Geometry: final body of the model. Coordinates: model frame, mm. Give positions to 0.01 mm unless a question says otherwise; leave off trailing zeros. Order: outer loops, then holes, each group sorted by start corner. A loop starts at its lowest first (then second) coordinate and runs counter-clockwise, first axis right, second up. Notation, with made-up numbers: (24, 15) -> (35, 15) arc R28 cw to (35, 45) -> close; hole circle Ø7 at (73.5, 53). An arc over 180 degrees is marked (long way). One line per question, with ' | ' between items.
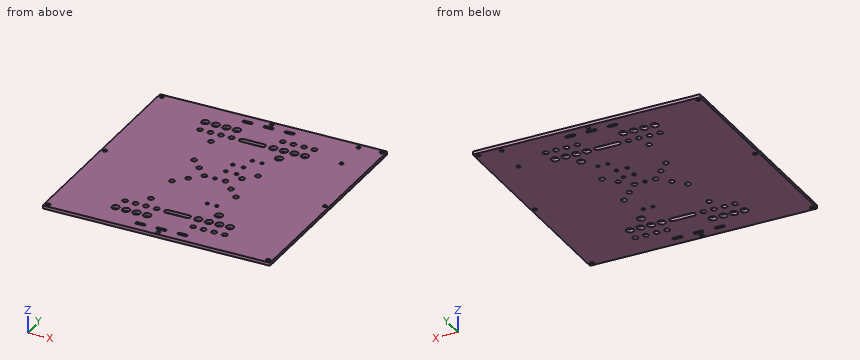
from build123d import *

# Parameters (mm, degrees)
SKETCH1_R           = 1.8
SKETCH1_R_2         = 2.5
SKETCH1_R_3         = 3.6
SKETCH1_R_4         = 1.57
SKETCH1_R_5         = 1.75
BOSS_EXTRUDE1_DEPTH = 3


with BuildPart() as part:
    # Sketch1 → Boss-Extrude1 (new body)
    with BuildSketch(Plane.XY):
        with BuildLine():
            Line((-107.125, -108), (107.125, -108))
            ThreePointArc((107.125, -108), (107.743718434, -107.743718434), (108, -107.125))
            Line((108, -107.125), (108, 107.125))
            ThreePointArc((108, 107.125), (107.743718434, 107.743718434), (107.125, 108))
            Line((107.125, 108), (-107.125, 108))
            ThreePointArc((-107.125, 108), (-107.743718434, 107.743718434), (-108, 107.125))
            Line((-108, 107.125), (-108, -107.125))
            ThreePointArc((-108, -107.125), (-107.743718434, -107.743718434), (-107.125, -108))
        make_face()
        with Locations((-104.5, -104.5)):
            Circle(SKETCH1_R, mode=Mode.SUBTRACT)
        with Locations((104.5, -104.5)):
            Circle(SKETCH1_R, mode=Mode.SUBTRACT)
        with Locations((-104.5, 104.5)):
            Circle(SKETCH1_R, mode=Mode.SUBTRACT)
        with Locations((104.5, 104.5)):
            Circle(SKETCH1_R, mode=Mode.SUBTRACT)
        with Locations((-49.85, -69)):
            Circle(SKETCH1_R_2, mode=Mode.SUBTRACT)
        with Locations((-39.85, -69)):
            Circle(SKETCH1_R_2, mode=Mode.SUBTRACT)
        with Locations((-29.85, -69)):
            Circle(SKETCH1_R_2, mode=Mode.SUBTRACT)
        with Locations((-19.855, -69)):
            Circle(SKETCH1_R_2, mode=Mode.SUBTRACT)
        with Locations((49.85, -69)):
            Circle(SKETCH1_R_3, mode=Mode.SUBTRACT)
        with Locations((39.85, -69)):
            Circle(SKETCH1_R_3, mode=Mode.SUBTRACT)
        with Locations((29.85, -69)):
            Circle(SKETCH1_R_3, mode=Mode.SUBTRACT)
        with Locations((19.855, -69)):
            Circle(SKETCH1_R_3, mode=Mode.SUBTRACT)
        with Locations((0, -104.5)):
            Circle(SKETCH1_R, mode=Mode.SUBTRACT)
        with Locations((0, 104.5)):
            Circle(SKETCH1_R, mode=Mode.SUBTRACT)
        with Locations((49.85, 69)):
            Circle(SKETCH1_R_3, mode=Mode.SUBTRACT)
        with Locations((39.85, 69)):
            Circle(SKETCH1_R_3, mode=Mode.SUBTRACT)
        with Locations((29.85, 69)):
            Circle(SKETCH1_R_3, mode=Mode.SUBTRACT)
        with Locations((19.855, 69)):
            Circle(SKETCH1_R_3, mode=Mode.SUBTRACT)
        with Locations((-19.855, 69)):
            Circle(SKETCH1_R_2, mode=Mode.SUBTRACT)
        with Locations((-29.85, 69)):
            Circle(SKETCH1_R_2, mode=Mode.SUBTRACT)
        with Locations((-39.85, 69)):
            Circle(SKETCH1_R_2, mode=Mode.SUBTRACT)
        with Locations((-49.85, 69)):
            Circle(SKETCH1_R_2, mode=Mode.SUBTRACT)
        with Locations((-104.5, 0)):
            Circle(SKETCH1_R, mode=Mode.SUBTRACT)
        with Locations((104.5, 0)):
            Circle(SKETCH1_R, mode=Mode.SUBTRACT)
        with Locations((-51.83, -82.65)):
            Circle(SKETCH1_R_3, mode=Mode.SUBTRACT)
        with Locations((-41.83, -82.65)):
            Circle(SKETCH1_R_3, mode=Mode.SUBTRACT)
        with Locations((-31.83, -82.65)):
            Circle(SKETCH1_R_3, mode=Mode.SUBTRACT)
        with Locations((-21.835, -82.65)):
            Circle(SKETCH1_R_3, mode=Mode.SUBTRACT)
        with Locations((51.83, -82.65)):
            Circle(SKETCH1_R_2, mode=Mode.SUBTRACT)
        with Locations((41.83, -82.65)):
            Circle(SKETCH1_R_2, mode=Mode.SUBTRACT)
        with Locations((31.83, -82.65)):
            Circle(SKETCH1_R_2, mode=Mode.SUBTRACT)
        with Locations((21.835, -82.65)):
            Circle(SKETCH1_R_2, mode=Mode.SUBTRACT)
        with Locations((-51.83, 82.65)):
            Circle(SKETCH1_R_3, mode=Mode.SUBTRACT)
        with Locations((-41.83, 82.65)):
            Circle(SKETCH1_R_3, mode=Mode.SUBTRACT)
        with Locations((-31.83, 82.65)):
            Circle(SKETCH1_R_3, mode=Mode.SUBTRACT)
        with Locations((-21.835, 82.65)):
            Circle(SKETCH1_R_3, mode=Mode.SUBTRACT)
        with Locations((51.83, 82.65)):
            Circle(SKETCH1_R_2, mode=Mode.SUBTRACT)
        with Locations((41.83, 82.65)):
            Circle(SKETCH1_R_2, mode=Mode.SUBTRACT)
        with Locations((31.83, 82.65)):
            Circle(SKETCH1_R_2, mode=Mode.SUBTRACT)
        with Locations((21.835, 82.65)):
            Circle(SKETCH1_R_2, mode=Mode.SUBTRACT)
        with Locations((83, 103)):
            Circle(SKETCH1_R, mode=Mode.SUBTRACT)
        with Locations((83, 72)):
            Circle(SKETCH1_R, mode=Mode.SUBTRACT)
        with Locations((-32.3, -55.35)):
            Circle(SKETCH1_R_2, mode=Mode.SUBTRACT)
        with Locations((32.3, -55.35)):
            Circle(SKETCH1_R_3, mode=Mode.SUBTRACT)
        with Locations((32.3, 55.35)):
            Circle(SKETCH1_R_3, mode=Mode.SUBTRACT)
        with Locations((-32.3, 55.35)):
            Circle(SKETCH1_R_2, mode=Mode.SUBTRACT)
        with Locations((14, -41.57)):
            Circle(SKETCH1_R_4, mode=Mode.SUBTRACT)
        with Locations((23.12, -41.57)):
            Circle(SKETCH1_R_4, mode=Mode.SUBTRACT)
        with Locations((23.12, 41.57)):
            Circle(SKETCH1_R_4, mode=Mode.SUBTRACT)
        with Locations((14, 41.57)):
            Circle(SKETCH1_R_4, mode=Mode.SUBTRACT)
        Circle(SKETCH1_R, mode=Mode.SUBTRACT)
        with Locations((-10, 0)):
            Circle(SKETCH1_R_2, mode=Mode.SUBTRACT)
        with Locations((10, 0)):
            Circle(SKETCH1_R_2, mode=Mode.SUBTRACT)
        with Locations((-20.32, 10.16)):
            Circle(SKETCH1_R_2, mode=Mode.SUBTRACT)
        with Locations((-30.32, 20.32)):
            Circle(SKETCH1_R_2, mode=Mode.SUBTRACT)
        with Locations((30.32, 20.32)):
            Circle(SKETCH1_R_2, mode=Mode.SUBTRACT)
        with Locations((20.32, 10.16)):
            Circle(SKETCH1_R_2, mode=Mode.SUBTRACT)
        with Locations((30.32, -20.32)):
            Circle(SKETCH1_R_2, mode=Mode.SUBTRACT)
        with Locations((20.32, -10.16)):
            Circle(SKETCH1_R_2, mode=Mode.SUBTRACT)
        with Locations((-20.32, -10.16)):
            Circle(SKETCH1_R_2, mode=Mode.SUBTRACT)
        with Locations((-30.32, -20.32)):
            Circle(SKETCH1_R_2, mode=Mode.SUBTRACT)
        with Locations((2.5, 28)):
            Circle(SKETCH1_R_5, mode=Mode.SUBTRACT)
        with Locations((12.64, 28)):
            Circle(SKETCH1_R_5, mode=Mode.SUBTRACT)
        with Locations((2.5, 15.17)):
            Circle(SKETCH1_R_5, mode=Mode.SUBTRACT)
        with Locations((12.64, 15.17)):
            Circle(SKETCH1_R_5, mode=Mode.SUBTRACT)
        with BuildLine():
            Line((-3.25, -97.12), (3.25, -97.12))
            ThreePointArc((3.25, -97.12), (4.75, -98.62), (3.25, -100.12))
            Line((3.25, -100.12), (-3.25, -100.12))
            ThreePointArc((-3.25, -100.12), (-4.75, -98.62), (-3.25, -97.12))
        make_face(mode=Mode.SUBTRACT)
        with BuildLine():
            Line((-23.25, -97.12), (-16.75, -97.12))
            ThreePointArc((-16.75, -97.12), (-15.25, -98.62), (-16.75, -100.12))
            Line((-16.75, -100.12), (-23.25, -100.12))
            ThreePointArc((-23.25, -100.12), (-24.75, -98.62), (-23.25, -97.12))
        make_face(mode=Mode.SUBTRACT)
        with BuildLine():
            Line((23.25, -97.12), (16.75, -97.12))
            ThreePointArc((16.75, -97.12), (15.25, -98.62), (16.75, -100.12))
            Line((16.75, -100.12), (23.25, -100.12))
            ThreePointArc((23.25, -100.12), (24.75, -98.62), (23.25, -97.12))
        make_face(mode=Mode.SUBTRACT)
        with BuildLine():
            Line((-3.25, 97.12), (3.25, 97.12))
            ThreePointArc((3.25, 97.12), (4.75, 98.62), (3.25, 100.12))
            Line((3.25, 100.12), (-3.25, 100.12))
            ThreePointArc((-3.25, 100.12), (-4.75, 98.62), (-3.25, 97.12))
        make_face(mode=Mode.SUBTRACT)
        with BuildLine():
            Line((23.25, 97.12), (16.75, 97.12))
            ThreePointArc((16.75, 97.12), (15.25, 98.62), (16.75, 100.12))
            Line((16.75, 100.12), (23.25, 100.12))
            ThreePointArc((23.25, 100.12), (24.75, 98.62), (23.25, 97.12))
        make_face(mode=Mode.SUBTRACT)
        with BuildLine():
            Line((-23.25, 97.12), (-16.75, 97.12))
            ThreePointArc((-16.75, 97.12), (-15.25, 98.62), (-16.75, 100.12))
            Line((-16.75, 100.12), (-23.25, 100.12))
            ThreePointArc((-23.25, 100.12), (-24.75, 98.62), (-23.25, 97.12))
        make_face(mode=Mode.SUBTRACT)
        with BuildLine():
            Line((-10, -66.5), (10, -66.5))
            ThreePointArc((10, -66.5), (12.5, -69), (10, -71.5))
            Line((10, -71.5), (-10, -71.5))
            ThreePointArc((-10, -71.5), (-12.5, -69), (-10, -66.5))
        make_face(mode=Mode.SUBTRACT)
        with BuildLine():
            Line((-10, 71.5), (10, 71.5))
            ThreePointArc((10, 71.5), (12.5, 69), (10, 66.5))
            Line((10, 66.5), (-10, 66.5))
            ThreePointArc((-10, 66.5), (-12.5, 69), (-10, 71.5))
        make_face(mode=Mode.SUBTRACT)
    extrude(amount=BOSS_EXTRUDE1_DEPTH)


solid = part.part
1) Material intervals for probe 1 along Y at (x, z) = (-2.5, 1); probe 2 along Y at (x, z) = (-9.5, 0.85); probe 3 along X at (y, z) = (22, 2.45), sorted ascending. Write a range as from..to.
Check result:
probe 1: y = -108..-100.12, -97.12..-71.5, -66.5..66.5, 71.5..97.12, 100.12..108 | probe 2: y = -108..-71.5, -66.5..-2.45, 2.45..66.5, 71.5..108 | probe 3: x = -108..-32.17, -28.47..28.47, 32.17..108
2) Section A-A on y = 10.16. Return loops of the section in (x, z), plus the area to 3 significant figures.
Check result:
outline: (-108, 0) -> (-22.82, 0) -> (-22.82, 3) -> (-108, 3) -> close; (-17.82, 0) -> (17.82, 0) -> (17.82, 3) -> (-17.82, 3) -> close; (22.82, 0) -> (108, 0) -> (108, 3) -> (22.82, 3) -> close | area: 618 mm^2
3) Contact query for a flat-ended pin moving along its axis: pin 1 Ø4 at (x, y) = (51.83, -82.65) entering from -Z. Output: stop coordinate, or through.
Check result:
pin 1: passes through
4) Section B-B on y = 82.65. Count the separate pieces of the cut face and the enclosed holes in it, plus the area to 3 significant figures.
Check result:
separate pieces: 9 | enclosed holes: 0 | area: 502 mm^2
